```python
from build123d import *

# Parameters (mm, degrees)
F0_W     = 40
F0_H     = 40
F1_DEPTH = 30
F2_W     = 10
F2_H     = 10
F3_DEPTH = 40
F5_DEPTH = 20
F6_W     = 20
F6_H     = 10
F7_DEPTH = 10
F9_DEPTH = 30


with BuildPart() as f1:
    # F0 (on Top) → F1 (new body)
    with BuildSketch(Plane.XY):
        Rectangle(F0_W, F0_H)
    extrude(amount=F1_DEPTH)

    # F2 (on face) → F3 (cut)
    with BuildSketch(Plane.XY.offset(30)):
        with Locations((-15, 15)):
            Rectangle(F2_W, F2_H)
    extrude(amount=-F3_DEPTH, mode=Mode.SUBTRACT)

    # F4 (on face) → F5 (cut)
    with BuildSketch(Plane.YZ.offset(20)):
        Polygon((10, 30), (-20, 30), (-20, 10), (-10, 10), (10, 20), align=None)
    extrude(amount=-F5_DEPTH, mode=Mode.SUBTRACT)

    # F6 (on face) → F7 (cut)
    with BuildSketch(Plane.YZ):
        with Locations((-10, 25)):
            Rectangle(F6_W, F6_H)
    extrude(amount=-F7_DEPTH, mode=Mode.SUBTRACT)

    # F8 (on face) → F9 (cut)
    with BuildSketch(Plane.XZ.offset(20)):
        Polygon((10, 10), (10, 30), (0, 30), (0, 20), (0, 10), align=None)
    extrude(amount=-F9_DEPTH, mode=Mode.SUBTRACT)


solid = f1.part
```
CAD build for the part. Positions are in the model's coordinates, mm. A direction names the side the tool comes from. Round coordinates to 2 decimals unless told otherwise and drop trailing zeros. Order: outer loops, then holes, each group sorted by start corner. A loop starts at its lowest first (then second) coordinate and runs counter-clockwise, first axis right, second up.
Q1. Drop flat-ended pins along their axis: pin 1 (8 mm diameter, centred on x = -14.5, z = 13, fed in from +Y); pin 2 (5 mm diameter, centred on y = -6, z = 24, fed in from +X); pin 3 (1 mm diameter, centred on x = 8.5, y = -8, fed in from +Z). Give the stop position or say it passes through.
Q2. Slice it at A-A (z = 14). Write the cut outline in (x, y), and give its area (3 significant figures).
Q3. Slice it at B-B (y = 2.5). Write the cut outline in (x, z), and give its area (4 significant figures).
Q4. Wall check: L1, parallel to X at y = 7.5, z = 17; L2, parallel to X at y = -9, z = 23.25; L3, parallel to Z at x = -4, y = -13. Give the ranges that are in metal, low to high.
Q5. Two-plate mould, pull along X, no slides. Class faces 6 (the flat face through (-5, -20, 11)), 7 (the flat face through (-10, -10, 25)), 8 (the flat face through (8, -9, 10)): pulls with the +X half, pulls with the -X half, needs draft (parallel to the pull), parting line crosses it, or undercut.
Q6. Which spindle directions (+Z, -Z, +X, -X, +Y, -Y) get a long thin tool onto all of the face, cutting with end or side? Do faces 1 (the flat face through (-5, 0, 25)), 2 (the flat face through (-10, 15, 15)), 3 (the flat face through (0, -2, 18)), 4 (the flat face through (-5, 5, 30)), 5 (the flat face through (-20, -5, 15)). Say none if no direction does.
Q7. Slice it at C-C (x = -3). Write the cut outline in (y, z), and give its area (3 significant figures).
Q8. Slice it at D-D (y = -1.5). Write the cut outline in (x, z).
Results below:
1. pin 1: stops at y = 10
1. pin 2: stops at x = -10
1. pin 3: stops at z = 10
2. outline: (-20, -20) - (0, -20) - (0, 10) - (10, 10) - (10, -2) - (20, -2) - (20, 20) - (-10, 20) - (-10, 10) - (-20, 10) - close
2. area: 1,020 mm2
3. outline: (-20, 0) - (20, 0) - (20, 16.25) - (10, 16.25) - (10, 10) - (0, 10) - (0, 30) - (-20, 30) - close
3. area: 862.5 mm2
4. L1: x = -20 to 0, 10 to 20
4. L2: x = -20 to -10
4. L3: z = 0 to 20
5. face 6: needs draft
5. face 7: pulls with the +X half
5. face 8: undercut
6. face 1: +Z, +X, -Y
6. face 2: +Z, -Z, -X, +Y
6. face 3: +Z, -Y
6. face 4: +Z, +X, -X, +Y, -Y
6. face 5: +Z, -Z, -X, +Y, -Y
7. outline: (-20, 0) - (20, 0) - (20, 30) - (0, 30) - (0, 20) - (-20, 20) - close
7. area: 1,000 mm2
8. outline: (-20, 0) - (20, 0) - (20, 14.25) - (10, 14.25) - (10, 10) - (0, 10) - (0, 20) - (-10, 20) - (-10, 30) - (-20, 30) - close
